```python
from build123d import *

# Parameters (mm, degrees)
SKETCH1_W               = 5
SKETCH1_H               = 10
BOSS_EXTRUDE1_DEPTH     = 1.5
SKETCH2_W               = 5
SKETCH2_H               = 11.5
BOSS_EXTRUDE2_DEPTH     = 1.5
SKETCH3_R               = 1.5
CUT_EXTRUDE1_DEPTH      = 1.5
CUT_EXTRUDE1_DEPTH_BACK = 10
SKETCH4_R               = 1.5
CUT_EXTRUDE2_DEPTH      = 10
CUT_EXTRUDE2_DEPTH_BACK = 10
FILLET1_R               = 1
FILLET2_R               = 1


with BuildPart() as part:
    # Sketch1 → Boss-Extrude1 (new body)
    with BuildSketch(Plane(origin=(0, 0, 0), x_dir=(1, 0, 0), z_dir=(0, 1, 0))):
        with Locations((2.5, 5)):
            Rectangle(SKETCH1_W, SKETCH1_H)
    extrude(amount=BOSS_EXTRUDE1_DEPTH)

    # Sketch2 → Boss-Extrude2 (add)
    with BuildSketch(Plane.XY):
        with Locations((2.5, 5.75)):
            Rectangle(SKETCH2_W, SKETCH2_H)
    extrude(amount=BOSS_EXTRUDE2_DEPTH)

    # Sketch3 → Cut-Extrude1 (cut, two sides)
    with BuildSketch(Plane(origin=(0, 1.5, 0), x_dir=(1, 0, 0), z_dir=(0, 1, 0))) as cut_extrude1_sk:
        with Locations((2.5, 5)):
            Circle(SKETCH3_R)
    extrude(amount=CUT_EXTRUDE1_DEPTH, mode=Mode.SUBTRACT)
    extrude(cut_extrude1_sk.sketch, amount=-CUT_EXTRUDE1_DEPTH_BACK, mode=Mode.SUBTRACT)

    # Sketch4 → Cut-Extrude2 (cut, two sides)
    with BuildSketch(Plane(origin=(0, 0, 0), x_dir=(-1, 0, 0), z_dir=(0, 0, -1))) as cut_extrude2_sk:
        with Locations((-2.5, 6.5)):
            Circle(SKETCH4_R)
    extrude(amount=CUT_EXTRUDE2_DEPTH, mode=Mode.SUBTRACT)
    extrude(cut_extrude2_sk.sketch, amount=-CUT_EXTRUDE2_DEPTH_BACK, mode=Mode.SUBTRACT)

    # Fillet1
    fillet1_edges = [part.edges().sort_by_distance(p)[0] for p in [
        (2.5, 1.5, 0),
    ]]
    fillet(fillet1_edges, radius=FILLET1_R)

    # Fillet2
    fillet2_edges = [part.edges().sort_by_distance(p)[0] for p in [
        (2.5, 0, 1.5),
    ]]
    fillet(fillet2_edges, radius=FILLET2_R)


solid = part.part
```
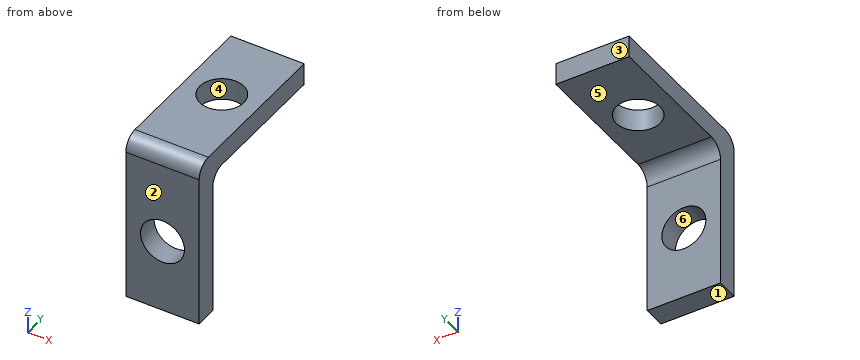
For this review, take the finished solid that the model builds, in its own axes (mm). Face numbers are marked on the shaded views. A direction names the side the tool comes from. Give positions to 0.01 mm unless a question says otherwise; leave off trailing zeros. Write each loop counter-clockwise with the first axis right and the second up, starting at its lowest first coordinate (ties: lowest second). Pieces come first, ordered by that corner, then holes.
Item 1: Take a section at D-D (x = 0.7). Give the boundary of the cut face in (y, z).
Item 2: Take a section at A-A (z = -5). Give the boundary of the cut face in (x, y), and give its area (3 significant figures).
Item 3: Take a section at C-C (x = 2.5). Give the boundary of the cut face in (y, z), and give its area (4 significant figures).
Item 4: The part is to be moulded in two halves that separate along Y. For the marked faces 1, 2, 3 and 4, say which applies: +Y half, -Y half, draft (parallel to the pull), parting line (faces both ways), or undercut.
Item 5: Insertion check: P1, Ø2, axis at x = 1.5, y = 3, coming from the -Z side; P2, Ø2.5, axis at x = 2, z = -4.5, coming from the +Y side; P3, Ø1, axis at x = 3.5, y = 5.5, coming from the -Z side. Each pin has a flat end and moves straight along its axis. Give the tip position at first contact, or say it passes through.
Item 6: Machinability: for the marked faces 5 and 6, which of the approach directions +Z, -Z, +X, -X, +Y, -Y give a long, thin tool a straight path to every point of the face, cutting with its end or side? Answer none if there is none.
Item 7: Wall thickness on probe 1 along X at (y, z) = (0.65, -5); probe 2 along Y at (x, z) = (4.5, -7): over which ranges is each line inside the solid? List them lowest first.
Established:
1. outline: (0, -10) - (1.5, -10) - (1.5, -1) arc R1 cw to (2.5, 0) - (11.5, 0) - (11.5, 1.5) - (1, 1.5) arc R1 ccw to (0, 0.5) - close
2. outline: (0, 0) - (1, 0) - (1, 1.5) - (0, 1.5) - close; (4, 0) - (5, 0) - (5, 1.5) - (4, 1.5) - close
2. area: 3.00 mm2
3. outline: (0, -10) - (1.5, -10) - (1.5, -6.5) - (0, -6.5) - close; (0, -3.5) - (1.5, -3.5) - (1.5, -1) arc R1 cw to (2.5, 0) - (5, 0) - (5, 1.5) - (1, 1.5) arc R1 ccw to (0, 0.5) - close; (8, 0) - (11.5, 0) - (11.5, 1.5) - (8, 1.5) - close
3. area: 23.25 mm2
4. face 1: draft
4. face 2: -Y half
4. face 3: +Y half
4. face 4: undercut
5. P1: stops at z = -0.13
5. P2: stops at y = 1.5
5. P3: stops at z = 0
6. face 5: -Z, +X, -X, +Y
6. face 6: +Y, -Y
7. probe 1: x = 0 to 1, 4 to 5
7. probe 2: y = 0 to 1.5
